```python
from build123d import *

# Parameters (mm, degrees)
SKETCH2_W           = 19
SKETCH2_H           = 35
BOSS_EXTRUDE1_DEPTH = 5
SKETCH3_W           = 5
SKETCH3_H           = 2.65
BOSS_EXTRUDE2_DEPTH = 13.5
SKETCH3_2_W         = 5
SKETCH3_2_H         = 2.65
BOSS_EXTRUDE3_DEPTH = 13.5
SKETCH4_R           = 5.075
CUT_EXTRUDE1_DEPTH  = 6
SKETCH5_R           = 10.5
CUT_EXTRUDE2_DEPTH  = 0.5
SKETCH7_W           = 18
SKETCH7_H           = 1.25
CUT_EXTRUDE3_DEPTH  = 22.2
SKETCH8_W           = 9
SKETCH8_H           = 2
CUT_EXTRUDE4_DEPTH  = 19
CUT_EXTRUDE5_DEPTH  = 1
SKETCH10_W          = 3.4
SKETCH10_H          = 4
CUT_EXTRUDE6_DEPTH  = 1


with BuildPart() as part:
    # Sketch2 → Boss-Extrude1 (new body)
    with BuildSketch(Plane.XY):
        with Locations((-7.329268293, 8.069105691)):
            Rectangle(SKETCH2_W, SKETCH2_H)
    extrude(amount=BOSS_EXTRUDE1_DEPTH)

    # Sketch3 → Boss-Extrude2 (add)
    with BuildSketch(Plane(origin=(-7.329268293, 0, 0), x_dir=(0, 0, -1), z_dir=(1, 0, 0))):
        with Locations((-2.5, 18.344105691)):
            Rectangle(SKETCH3_W, SKETCH3_H)
        with Locations((-2.5, 3.494105691)):
            Rectangle(SKETCH3_W, SKETCH3_H)
    extrude(amount=BOSS_EXTRUDE2_DEPTH)

    # Sketch3_2 → Boss-Extrude3 (add)
    with BuildSketch(Plane(origin=(-7.329268293, 0, 0), x_dir=(0, 0, -1), z_dir=(1, 0, 0))):
        with Locations((-2.5, 18.344105691)):
            Rectangle(SKETCH3_2_W, SKETCH3_2_H)
        with Locations((-2.5, 3.494105691)):
            Rectangle(SKETCH3_2_W, SKETCH3_2_H)
    extrude(amount=-BOSS_EXTRUDE3_DEPTH)

    # Sketch4 → Cut-Extrude1 (cut, through all)
    with BuildSketch(Plane.XY.offset(5)):
        with Locations((-7.329268293, -2.173702028)):
            Circle(SKETCH4_R)
    extrude(amount=-CUT_EXTRUDE1_DEPTH, mode=Mode.SUBTRACT)

    # Sketch5 → Cut-Extrude2 (cut)
    with BuildSketch(Plane.XY.offset(5)):
        with Locations((-7.329268293, -2.173702028)):
            Circle(SKETCH5_R)
    extrude(amount=-CUT_EXTRUDE2_DEPTH, mode=Mode.SUBTRACT)

    # Sketch7 → Cut-Extrude3 (cut)
    with BuildSketch(Plane(origin=(0, 25.569105691, 0), x_dir=(1, 0, 0), z_dir=(0, 1, 0))):
        with Locations((-7.329268293, -2.625)):
            Rectangle(SKETCH7_W, SKETCH7_H)
    extrude(amount=-CUT_EXTRUDE3_DEPTH, mode=Mode.SUBTRACT)

    # Sketch8 → Cut-Extrude4 (cut)
    with BuildSketch(Plane(origin=(0, 25.569105691, 0), x_dir=(1, 0, 0), z_dir=(0, 1, 0))):
        with Locations((-7.329268293, -1)):
            Rectangle(SKETCH8_W, SKETCH8_H)
    extrude(amount=-CUT_EXTRUDE4_DEPTH, mode=Mode.SUBTRACT)

    # Sketch9 → Cut-Extrude5 (cut)
    with BuildSketch(Plane.XZ.offset(-2.169105691)):
        Polygon((-20.529268293, 4.5), (-17.129268293, 4.5), (-17.129268293, 3.5), (-17.129268293, 1.5), (-17.129268293, 0.5), (-20.529268293, 0.5), (-20.529268293, 1.5), (-20.529268293, 3.5), align=None)
        Polygon((2.470731707, 4.5), (5.870731707, 4.5), (5.870731707, 3.5), (5.870731707, 1.5), (5.870731707, 0.5), (2.470731707, 0.5), (2.470731707, 1.5), (2.470731707, 3.5), align=None)
    extrude(amount=-CUT_EXTRUDE5_DEPTH, mode=Mode.SUBTRACT)

    # Sketch10 → Cut-Extrude6 (cut)
    with BuildSketch(Plane.XZ.offset(-17.019105691)):
        with Locations((-18.829268293, 2.5)):
            Rectangle(SKETCH10_W, SKETCH10_H)
        with Locations((4.170731707, 2.5)):
            Rectangle(SKETCH10_W, SKETCH10_H)
    extrude(amount=-CUT_EXTRUDE6_DEPTH, mode=Mode.SUBTRACT)


solid = part.part
```
Work out the finished part from the listing and answer in its coordinate system (mm). A direction names the side the tool comes from. Give positions to 0.01 mm unless a question says otherwise; leave off trailing zeros. Write each loop counter-clockwise with the first axis right and the second up, starting at its lowest first coordinate (ties: lowest second). Pieces come first, ordered by that corner, then holes.
(1) Straight lines are drawn through the part: line 1 (X direction, y = 17.5, z = 1); line 2 (Z direction, x = -13.5, y = 14.5); line 3 (Y direction, x = -17, z = 4.4). For each, find the intervals that lie inside material, in ascending order.
Final values:
line 1: x = -20.83 to -20.53, -17.13 to -11.83, -2.83 to 2.47, 5.87 to 6.17
line 2: z = 0 to 2, 3.25 to 5
line 3: y = 2.17 to 4.82, 17.02 to 19.67
(2) The part is cut by section B-B on y = 10. Write down the section's boundary in (x, z).
Final values:
outline: (-16.83, 0) - (-11.83, 0) - (-11.83, 2) - (-16.33, 2) - (-16.33, 3.25) - (1.67, 3.25) - (1.67, 2) - (-2.83, 2) - (-2.83, 0) - (2.17, 0) - (2.17, 5) - (-16.83, 5) - close
(3) Flat-ended cylindrical pins translate along their axes: pin 1 Ø1.4 at (y, z) = (16, 2.5) entering from +X; pin 2 Ø1.2 at (x, z) = (4.5, 2.5) entering from +Y; pin 3 Ø2 at (x, z) = (-6.5, 1.5) entering from +Y; pin 4 Ø10 at (x, y) = (-11.5, 4.5) entering from +Z. Find the tip coordinate at first contact, or state that the pin passes through.
Final values:
pin 1: stops at x = 2.17
pin 2: stops at y = 19.67
pin 3: stops at y = 6.57
pin 4: stops at z = 5
(4) The part is cut by section C-C on y = -5. Write down the section's boundary in (x, z), plus the area to 3 significant figures.
Final values:
outline: (-16.83, 0) - (-11.54, 0) - (-11.54, 4.5) - (-16.83, 4.5) - close; (-3.11, 0) - (2.17, 0) - (2.17, 4.5) - (-3.11, 4.5) - close
area: 47.6 mm2
(5) Which of the six approach directions +Z, -Z, +X, -X, +Y, -Y give full straight-line access (tool end or side, diameter ignored) to faces 4 (the flat face through (4, 3, 0.5)), 5 (the flat face through (4, 19.669, 3)), 6 (the cylindrical face through (-7.161, 8.325, 4.754))?
Final values:
face 4: -Y
face 5: +Z, -Z, +X, +Y
face 6: +Z
(6) The part is cut by section D-D on x = -5.25. Write down the section's boundary in (y, z).
Final values:
outline: (-9.43, 0) - (-6.8, 0) - (-6.8, 4.5) - (-9.43, 4.5) - close; (2.46, 0) - (6.57, 0) - (6.57, 2) - (3.37, 2) - (3.37, 3.25) - (25.57, 3.25) - (25.57, 5) - (8.12, 5) - (8.12, 4.5) - (2.46, 4.5) - close
(7) The part is cut by section A-A on x = 4.5. Write down the section's boundary in (y, z).
Final values:
outline: (2.17, 0) - (4.82, 0) - (4.82, 5) - (2.17, 5) - (2.17, 4.5) - (3.17, 4.5) - (3.17, 0.5) - (2.17, 0.5) - close; (17.02, 0) - (19.67, 0) - (19.67, 5) - (17.02, 5) - (17.02, 4.5) - (18.02, 4.5) - (18.02, 0.5) - (17.02, 0.5) - close
(8) The mould has two halves that part along X. Classify faces 1 (the flat face through (-16.829, -4, 2)), 2 (the flat face through (5.871, 3, 2)), 3 (the flat face through (4, 4.819, 3)): pulls with the +X half, pulls with the -X half, needs draft (parallel to the pull), parting line crosses it, or undercut.
Final values:
face 1: pulls with the -X half
face 2: undercut
face 3: needs draft
